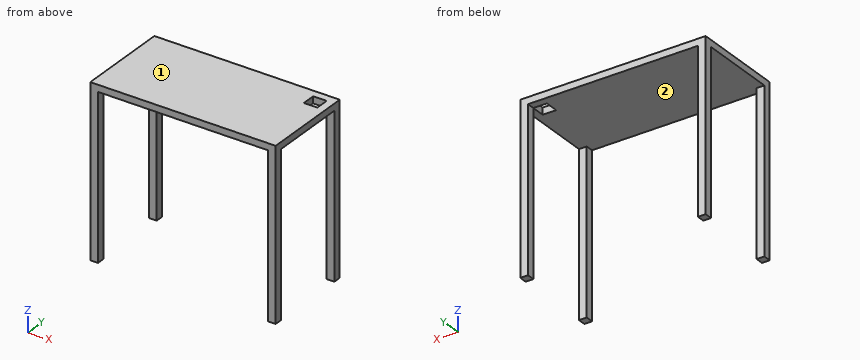
from build123d import *

# Parameters (mm, degrees)
F0_W     = 1219.2
F0_H     = 609.6
F1_DEPTH = 44.45
F2_W     = 88.9
F2_H     = 88.9
F3_DEPTH = 44.451
F4_W     = 50.8
F4_H     = 50.8
F5_DEPTH = 1066.8


with BuildPart() as f1:
    # F0 (on Top) → F1 (new body)
    with BuildSketch(Plane.XY):
        Rectangle(F0_W, F0_H)
    extrude(amount=F1_DEPTH)

    # F2 (on face) → F3 (cut, through all)
    with BuildSketch(Plane.XY.offset(44.45)):
        with Locations((514.35, 209.55)):
            Rectangle(F2_W, F2_H)
    extrude(amount=-F3_DEPTH, mode=Mode.SUBTRACT)

    # F4 (on face) → F5 (join)
    with BuildSketch(Plane(origin=(0, 0, 0), x_dir=(1, 0, 0), z_dir=(0, 0, -1))):
        with Locations((584.2, 279.4)):
            Rectangle(F4_W, F4_H)
        with Locations((-584.2, 279.4)):
            Rectangle(F4_W, F4_H)
        with Locations((-584.2, -279.4)):
            Rectangle(F4_W, F4_H)
        with Locations((584.2, -279.4)):
            Rectangle(F4_W, F4_H)
    extrude(amount=F5_DEPTH)


solid = f1.part
Verification items for the finished model (mm, model axes). Face numbers are marked on the shaded views. Coordinates: 2 decimals unless noted, no trailing zeros. Loops run counter-clockwise (first coordinate to the right, second up) from the corner with the lowest first, then second, coordinate; pieces in that order, holes last. Notation, with made-up numbers: (79, 46) -> (127, 46) arc R20 cw to (127, 65) -> close; hole circle Ø10 at (-0.5, -29). An arc over 180 degrees is marked (long way). Write each question's results on one line, items separated by ' | '.
Item 1: Mould release check, pull along X, two halves, no side actions. Record for the marked faces 1 and 2: +X half, -X half, draft (parallel to the pull), parting line (faces both ways), or undercut.
Found:
face 1: draft | face 2: undercut
Item 2: Section check D-D, the plane y = -111. Enter the section's corners in (x, z), plus the area to 3 significant figures.
Found:
outline: (-609.6, 0) -> (609.6, 0) -> (609.6, 44.45) -> (-609.6, 44.45) -> close | area: 54,200 mm2
Item 3: Section check C-C, the plane x = 484. Enter the section's corners in (y, z).
Found:
outline: (-304.8, 0) -> (165.1, 0) -> (165.1, 44.45) -> (-304.8, 44.45) -> close; (254, 0) -> (304.8, 0) -> (304.8, 44.45) -> (254, 44.45) -> close
Item 4: Material ranges on L1, parallel to X at y = 260, z = -109.5; L2, parallel to Z at x = 212, y = -115, recorded low to high.
Found:
L1: x = -609.6 to -558.8, 558.8 to 609.6 | L2: z = 0 to 44.45
Item 5: Section check A-A, the plane z = -560.5. Enter the section's corners in (x, y).
Found:
outline: (-609.6, -304.8) -> (-558.8, -304.8) -> (-558.8, -254) -> (-609.6, -254) -> close; (-609.6, 254) -> (-558.8, 254) -> (-558.8, 304.8) -> (-609.6, 304.8) -> close; (558.8, -304.8) -> (609.6, -304.8) -> (609.6, -254) -> (558.8, -254) -> close; (558.8, 254) -> (609.6, 254) -> (609.6, 304.8) -> (558.8, 304.8) -> close
Item 6: Section check B-B, the plane y = 223.5. Enter the section's corners in (x, z).
Found:
outline: (-609.6, 0) -> (469.9, 0) -> (469.9, 44.45) -> (-609.6, 44.45) -> close; (558.8, 0) -> (609.6, 0) -> (609.6, 44.45) -> (558.8, 44.45) -> close
Item 7: Gauge pin test, flat end, axial feed: pin 1 (5 mm diameter, centred on x = -255.5, y = -97, fed in from -Z). Record the tip position at first contact, or that the pin passes through.
Found:
pin 1: stops at z = 0
